For this review, take the finished solid that the model builds, in its own axes (mm). Coordinates: 2 decimals unless noted, no trailing zeros. Order: outer loops, then holes, each group sorted by start corner. A loop starts at its lowest first (then second) coordinate and runs counter-clockwise, first axis right, second up. Notation, with made-up numbers: (1.5, 82) -> (34.5, 82) arc R20 cw to (34.5, 89) -> close; hole circle Ø3 at (-36.75, 69). An arc over 180 degrees is marked (long way). Answer as a JSON object with one key per item and string values. Group by question number.
1) Add section D-D, the plane z = 70. Write out the cut boundary in (x, y).
2) Add section C-C, the plane z = -3. Write out the cut boundary in (x, y), then the cut area to 3 significant figures.
3) For pin 1 (5 mm diameter, centred on x = 474.5, y = 3, fed in from +Z); pin 2 (5 mm diameter, centred on y = 5.5, z = -60.5, fed in from +X); pin 3 (3 mm diameter, centred on y = 3, z = 81, fed in from -X), all flat-tipped, find the tip position at first contact; note any pin that passes through.
4) Add section B-B, the plane y = 5.75. Write out the cut boundary in (x, z).
5) Wall thickness on L1, parallel to X at y = 2.5, z = -36; L2, parallel to X at y = 9.25, z = -56.5; L3, parallel to X at y = 6.75, z = 81: over which ranges is each line inside the solid? List them lowest first.
6) Add section A-A, the plane z = -61. Write out the cut boundary in (x, y), then the cut area to 3 significant figures.
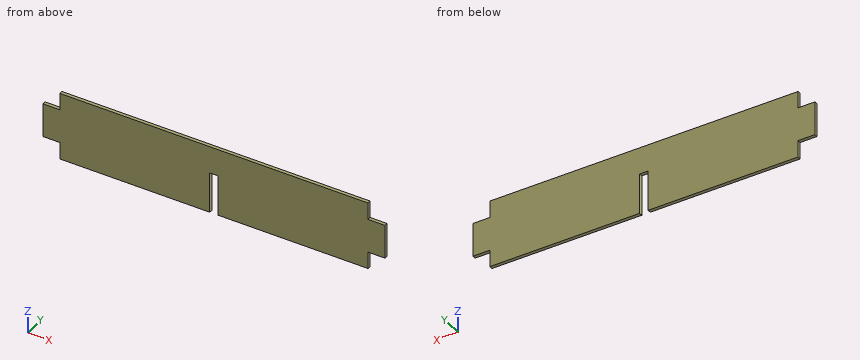
from build123d import *

# Parameters (mm, degrees)
SKETCH1_W               = 1010
SKETCH1_H               = 200
BOSS_EXTRUDE1_DEPTH     = 10
SKETCH2_W               = 50
SKETCH2_H               = 50
CUT_EXTRUDE1_DEPTH      = 10
MIRROR2_COPY_1_SKETCH_W = 50
MIRROR2_COPY_1_SKETCH_H = 50
MIRROR2_COPY_1_DEPTH    = 10
SKETCH3_W               = 25
SKETCH3_H               = 120
CUT_EXTRUDE3_DEPTH      = 10


with BuildPart() as part:
    # Sketch1 → Boss-Extrude1 (new body)
    with BuildSketch(Plane(origin=(0, 0, 0), x_dir=(1, 0, 0), z_dir=(0, 1, 0))):
        Rectangle(SKETCH1_W, SKETCH1_H)
    extrude(amount=BOSS_EXTRUDE1_DEPTH)

    # Sketch2 → Cut-Extrude1 (cut)
    with BuildSketch(Plane(origin=(0, 10, 0), x_dir=(1, 0, 0), z_dir=(0, 1, 0))):
        with Locations((-480, 75)):
            Rectangle(SKETCH2_W, SKETCH2_H)
    cut_extrude1 = extrude(amount=-CUT_EXTRUDE1_DEPTH, mode=Mode.SUBTRACT)

    # Mirror1: Cut-Extrude1 across plane
    add(cut_extrude1.mirror(Plane.XY), mode=Mode.SUBTRACT)

    # Mirror2: Cut-Extrude1 across plane
    add(cut_extrude1.mirror(Plane(origin=(0, 0, 0), x_dir=(0, 0, 1), z_dir=(1, 0, 0))), mode=Mode.SUBTRACT)

    # Mirror2 copy 1 sketch → Mirror2 copy 1 (cut)
    with BuildSketch(Plane(origin=(0, 10, 0), x_dir=(-1, 0, 0), z_dir=(0, 1, 0))):
        with Locations((-480, 75)):
            Rectangle(MIRROR2_COPY_1_SKETCH_W, MIRROR2_COPY_1_SKETCH_H)
    extrude(amount=-MIRROR2_COPY_1_DEPTH, mode=Mode.SUBTRACT)

    # Sketch3 → Cut-Extrude3 (cut)
    with BuildSketch(Plane(origin=(0, 0, 0), x_dir=(1, 0, 0), z_dir=(0, 1, 0))):
        with Locations((0, 40)):
            Rectangle(SKETCH3_W, SKETCH3_H)
    extrude(amount=CUT_EXTRUDE3_DEPTH, mode=Mode.SUBTRACT)


solid = part.part
Output values:
{
 "1": {"outline": "(-455, 0) -> (455, 0) -> (455, 10) -> (-455, 10) -> close"},
 "2": {"outline": "(-505, 0) -> (-12.5, 0) -> (-12.5, 10) -> (-505, 10) -> close; (12.5, 0) -> (505, 0) -> (505, 10) -> (12.5, 10) -> close", "area": "9,850 mm²"},
 "3": {"pin 1": "stops at z = 50", "pin 2": "stops at x = 455", "pin 3": "stops at x = -455"},
 "4": {"outline": "(-505, -50) -> (-455, -50) -> (-455, -100) -> (-12.5, -100) -> (-12.5, 20) -> (12.5, 20) -> (12.5, -100) -> (455, -100) -> (455, -50) -> (505, -50) -> (505, 50) -> (455, 50) -> (455, 100) -> (-455, 100) -> (-455, 50) -> (-505, 50) -> close"},
 "5": {"L1": "x = -505 to -12.5, 12.5 to 505", "L2": "x = -455 to -12.5, 12.5 to 455", "L3": "x = -455 to 455"},
 "6": {"outline": "(-455, 0) -> (-12.5, 0) -> (-12.5, 10) -> (-455, 10) -> close; (12.5, 0) -> (455, 0) -> (455, 10) -> (12.5, 10) -> close", "area": "8,850 mm²"}
}
